Verification items for this drawing (mm, ordinates from the low corner). Give positions to 0.01 mm unless a question says otherwise; leave off trailing zeros. Loops run counter-clockwise (first coordinate to the right, second up) from the corner with the lowest first, then second, coordinate; pieces in that order, holes last. Notation, with made-up numbers: M -35.5,-10 L 8.5,-10 A13 ccw 8.5,14 Z; hole C 47.5,78 d11. An arc over 180 degrees is marked long. Use one line per item in the form item = value.
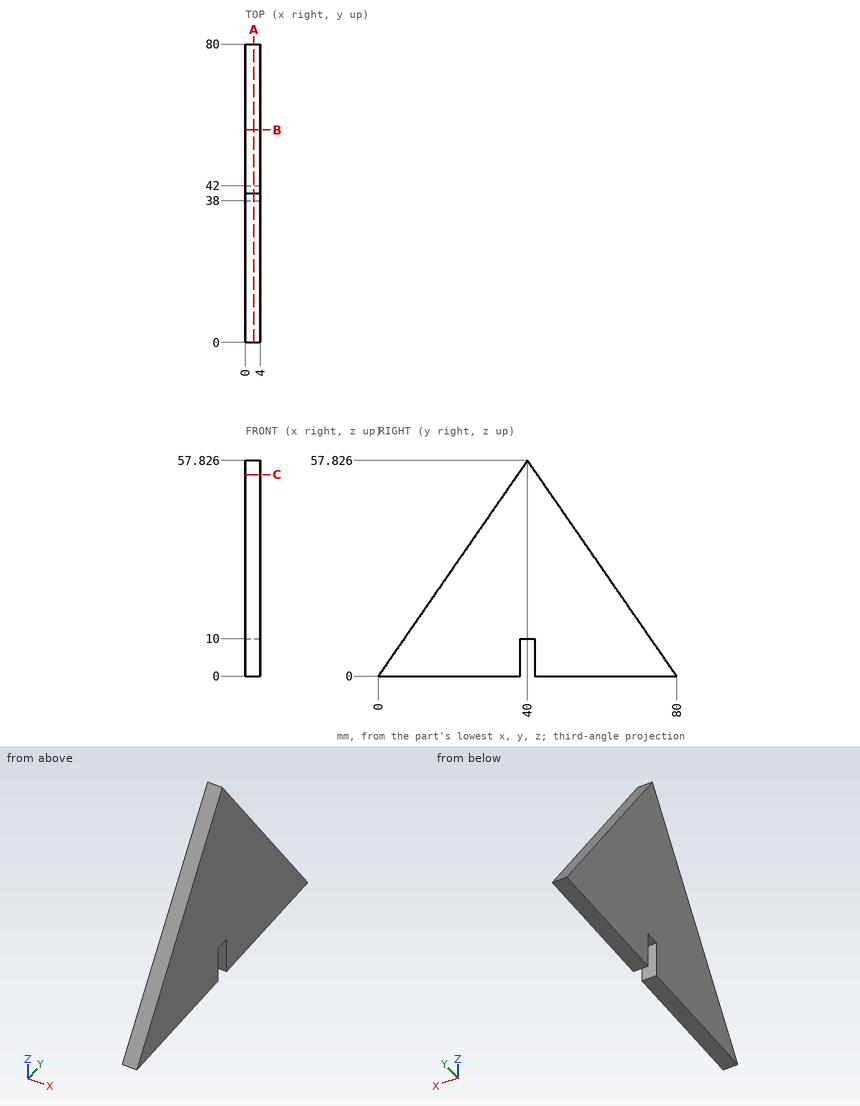
1) Section check B-B (y = 57). Record the cut outline in (x, z), then the cut area to 3 significant figures.
Evaluation:
outline = M 0,0 L 4,0 L 4,33.25 L 0,33.25 Z
area = 133 mm^2
2) Section check A-A (x = 2.25). Record the cut outline in (y, z), then the cut area to 3 significant figures.
Evaluation:
outline = M 0,0 L 38,0 L 38,10 L 42,10 L 42,0 L 80,0 L 40,57.83 Z
area = 2,270 mm^2
3) Section check C-C (z = 54). Record the cut outline in (x, y), then the cut area to 3 significant figures.
Evaluation:
outline = M 0,37.35 L 4,37.35 L 4,42.65 L 0,42.65 Z
area = 21.2 mm^2
4) Scan lines: line 1 (Y direction, x = 0.4, z = 7.5); line 2 (Y direction, x = 0.75, z = 3) (1 decimal); line 3 (Y direction, x = 0.75, z = 28.5). Record each from-to range of solid material in increasing order.
Evaluation:
line_1 = 5.19 to 38, 42 to 74.81
line_2 = 2.1 to 38, 42 to 77.9
line_3 = 19.71 to 60.29
5) Depth check by flat-ended pin: pin 1 Ø1.5 at (x, y) = (1.5, 44.5) entering from +Z (1 decimal); pin 2 Ø2 at (x, z) = (2, 4) entering from -Y (1 decimal). Enter the tip coordinate at first touch or a pass-through.
Evaluation:
pin_1 = 52.4
pin_2 = 2.1
